Check sheet for the modelled part. Datum: model origin and axes. Units: mm. Face numbers are marked on the shaded views. A direction names the side the tool comes from. Round coordinates to 2 decimals unless told otherwise and drop trailing zeros. Write each loop counter-clockwise with the first axis right and the second up, starting at its lowest first coordinate (ties: lowest second). Pieces come first, ordered by that corner, then holes.
Item 1: Section check A-A, the plane z = 12.7. Record the cut outline in (x, y), plus the area to 3 significant figures.
Item 2: Set-up check for the marked faces 1, 2 and 3: record each of +Z, -Z, +X, -X, +Y, -Y from which the full face is reachable in a straight line by a thin tool's end or side.
Item 3: Section check D-D, the plane y = 23. Record the cut outline in (x, z).
Item 4: Section check B-B, the plane y = 3.75. Record the cut outline in (x, z), plus the area to 3 significant figures.
Item 5: Material ranges on line 1 along Z through (x, y) = (25.4, 19.25); line 2 along X through (y, z) = (10, 11.5); line 3 along Y through (x, z) = (13.5, 18), recorded low to high.
Item 6: Depth check by flat-ended pin: pin 1 (6 mm diameter, centred on y = 21.5, z = 4, fed in from +X); pin 2 (12.5 mm diameter, centred on x = 23, z = 6.5, fed in from -Y); pin 3 (2 mm diameter, centred on x = 29.5, y = 11.5, fed in from +Z); pin 4 (6.5 mm diameter, centred on x = 4, z = 11, fed in from -Y). Enter the tip coordinate at first touch or a pass-through.
Item 7: Section check C-C, the plane x = 22.5. Record the cut outline in (y, z).
Item 8: Release check for a two-part mould opening along X. For the marked faces 4, 5, 6 and 7 record: pulls with the +X half, pulls with the -X half, needs draft (parallel to the pull), parting line crosses it, or undercut.
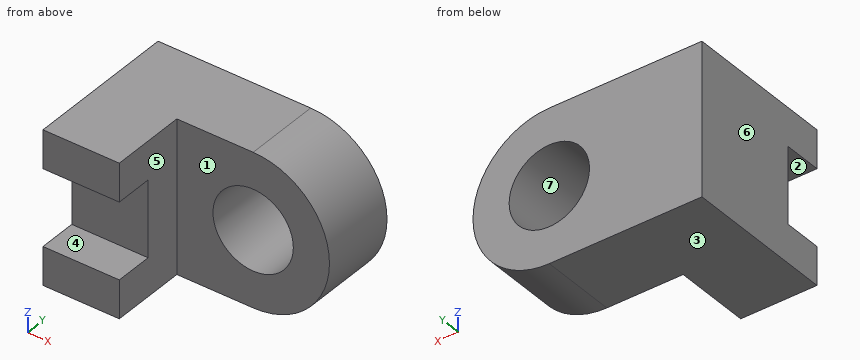
from build123d import *

# Parameters (mm, degrees)
F1_DEPTH = 25.4
F2_W     = 6.35
F2_H     = 12.7
F3_DEPTH = 25.4
F5_DEPTH = 12.7
F6_R     = 6.68714
F7_DEPTH = 25.4


with BuildPart() as f1:
    # F0 (on Top) → F1 (new body)
    with BuildSketch(Plane.XY):
        Polygon((0, 25.4), (0, 0), (12.7, 0), (12.7, 12.7), (25.4, 12.7), (25.4, 25.4), align=None)
    extrude(amount=F1_DEPTH)

    # F2 (on face) → F3 (cut)
    with BuildSketch(Plane.YZ.offset(12.7)):
        with Locations((3.175, 12.7)):
            Rectangle(F2_W, F2_H)
    extrude(amount=-F3_DEPTH, mode=Mode.SUBTRACT)

    # F4 (on face) → F5 (join)
    with BuildSketch(Plane.XZ.offset(-12.7)):
        with BuildLine():
            Line((25.4, 25.4), (25.4, 0))
            ThreePointArc((25.4, 0), (38.1, 12.7), (25.4, 25.4))
        make_face()
    extrude(amount=-F5_DEPTH)

    # F6 (on face) → F7 (cut)
    with BuildSketch(Plane.XZ.offset(-12.7)):
        with Locations((25.4, 12.7)):
            Circle(F6_R)
    extrude(amount=-F7_DEPTH, mode=Mode.SUBTRACT)


solid = f1.part
Values found:
1. outline: (0, 6.35) - (12.7, 6.35) - (12.7, 12.7) - (18.71, 12.7) - (18.71, 25.4) - (0, 25.4) - close; (32.09, 12.7) - (38.1, 12.7) - (38.1, 25.4) - (32.09, 25.4) - close
1. area: 395 mm2
2. face 1: +Z, -Z, +X, -Y
2. face 2: +X, -X, -Y
2. face 3: -Z, +X, -X, +Y, -Y
3. outline: (0, 0) - (25.4, 0) arc R12.7 ccw to (25.4, 25.4) - (0, 25.4) - close; hole circle Ø13.37 at (25.4, 12.7)
4. outline: (0, 0) - (12.7, 0) - (12.7, 6.35) - (0, 6.35) - close; (0, 19.05) - (12.7, 19.05) - (12.7, 25.4) - (0, 25.4) - close
4. area: 161 mm2
5. line 1: z = 0 to 6.01, 19.39 to 25.4
5. line 2: x = 0 to 12.7
5. line 3: y = 12.7 to 25.4
6. pin 1: stops at x = 36.75
6. pin 2: stops at y = 12.7
6. pin 3: passes through
6. pin 4: stops at y = 6.35
7. outline: (12.7, 0) - (25.4, 0) - (25.4, 6.67) - (12.7, 6.67) - close; (12.7, 18.73) - (25.4, 18.73) - (25.4, 25.4) - (12.7, 25.4) - close
8. face 4: needs draft
8. face 5: pulls with the +X half
8. face 6: pulls with the -X half
8. face 7: undercut
